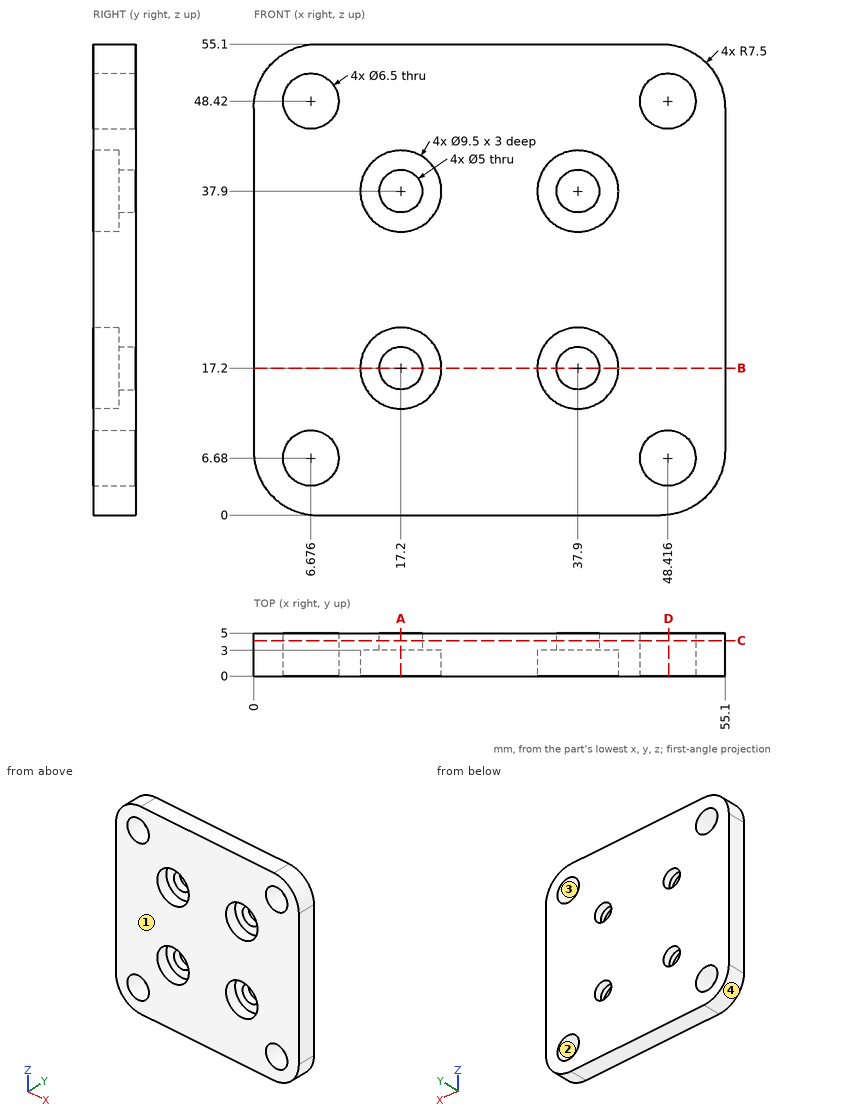
Here's the drawing with two shaded views (mm, measured from the low corner). I have some questions. Give positions to 0.01 mm unless a question says otherwise; leave off trailing zeros. Write each loop counter-clockwise with the first axis right and the second up, starting at its lowest first coordinate (ties: lowest second). Pieces come first, ordered by that corner, then holes. Notation, with made-up numbers: (-22, 64) - (37, 64) arc R19 ccw to (37, 98) - close; hole circle Ø2 at (59, -35.5). An arc over 180 degrees is marked (long way). Write item = value, one per line. Start each with the question number.
1. Please list where these lines run through material, in increasing order: line 1 (Z direction, x = 17, y = 3.65); line 2 (Z direction, x = 17.2, y = 0.7); line 3 (X direction, y = 0.75, z = 9.5).
2. For pin 1 (8.5 mm diameter, centred on x = 17.2, z = 37.9, fed in from -Y); pin 2 (6 mm diameter, centred on x = 48.42, z = 48.42, fed in from -Y), each with a flat end and sliding along its axis, tell me the tip position at first contact or that it passes through.
3. Imagine slicing it at C-C (y = 4.15). Count the separate pieces of the cut face and the enclosed holes in it, and give its area (3 significant figures).
4. Imagine slicing it at A-A (x = 17.2). Please give me the cut outline in (y, z).
5. Imagine slicing it at B-B (z = 17.2). Please give me the cut outline in (x, y).
6. Imagine slicing it at D-D (x = 48.5). Please give me the cut outline in (y, z).
7. Thinking about a two-plate mould opening in X: for the marked faces 1, 2, 3 and 4, which applies, released by +X, released by -X, zero draft, split by the parting line, or undercut?
Worked answers:
q1.line_1 = 0 to 14.71, 19.69 to 35.41, 40.39 to 55.1
q1.line_2 = 0 to 12.45, 21.95 to 33.15, 42.65 to 55.1
q1.line_3 = 0 to 5.06, 8.29 to 46.8, 50.03 to 55.1
q2.pin_1 = 3
q2.pin_2 = through
q3.separate_pieces = 1
q3.enclosed_holes = 8
q3.area = 2,780 mm2
q4.outline = (0, 0) - (5, 0) - (5, 14.7) - (3, 14.7) - (3, 12.45) - (0, 12.45) - close; (0, 21.95) - (3, 21.95) - (3, 19.7) - (5, 19.7) - (5, 35.4) - (3, 35.4) - (3, 33.15) - (0, 33.15) - close; (0, 42.65) - (3, 42.65) - (3, 40.4) - (5, 40.4) - (5, 55.1) - (0, 55.1) - close
q5.outline = (0, 0) - (12.45, 0) - (12.45, 3) - (14.7, 3) - (14.7, 5) - (0, 5) - close; (19.7, 3) - (21.95, 3) - (21.95, 0) - (33.15, 0) - (33.15, 3) - (35.4, 3) - (35.4, 5) - (19.7, 5) - close; (40.4, 3) - (42.65, 3) - (42.65, 0) - (55.1, 0) - (55.1, 5) - (40.4, 5) - close
q6.outline = (0, 0.05) - (5, 0.05) - (5, 3.43) - (0, 3.43) - close; (0, 9.93) - (5, 9.93) - (5, 45.17) - (0, 45.17) - close; (0, 51.67) - (5, 51.67) - (5, 55.05) - (0, 55.05) - close
q7.face_1 = zero draft
q7.face_2 = undercut
q7.face_3 = undercut
q7.face_4 = released by -X
